For this review, take the finished solid that the model builds, in its own axes (mm). Face numbers are marked on the shaded views. A direction names the side the tool comes from. Give positions to 0.01 mm unless a question says otherwise; leave off trailing zeros. Order: outer loops, then holes, each group sorted by start corner. A loop starts at its lowest first (then second) coordinate and runs counter-clockwise, first axis right, second up. Notation, with made-up numbers: (46.5, 26.5) -> (88.5, 26.5) arc R24 ccw to (88.5, 46.5) -> close; hole circle Ø2 at (33, 20.25). An arc over 180 degrees is marked (long way). One line per item, written item: value. Start each with the question number.
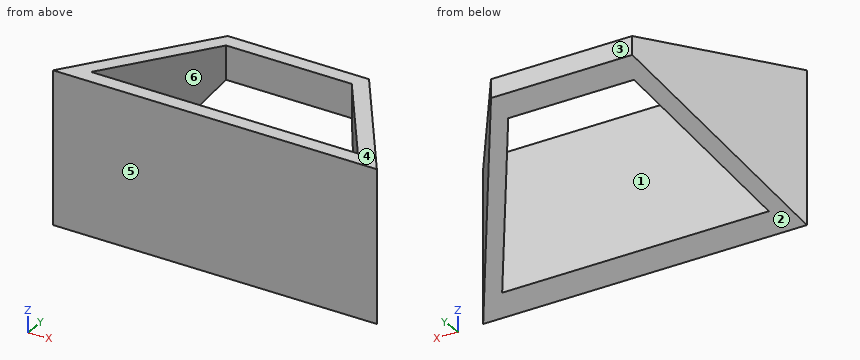
from build123d import *

# Parameters (mm, degrees)
F1_DEPTH      = 1000
F3_DEPTH      = 1091.0655359211
F3_DEPTH_BACK = 1091.0655359211


with BuildPart() as f1:
    # F0 (on Top) → F1 (new body)
    with BuildSketch(Plane.XY):
        Polygon((476.0241719385, 439.0613704803), (-476.0241719385, 439.0613704803), (-1091.0645359211, -439.0613704803), (1091.0645359211, -439.0613704803), align=None)
        Polygon((-898.9354640789, -339.0613704803), (-423.9758280615, 339.0613704803), (423.9758280615, 339.0613704803), (898.9354640789, -339.0613704803), align=None, mode=Mode.SUBTRACT)
    extrude(amount=F1_DEPTH)

    # F2 (on Right) → F3 (cut, two sides)
    with BuildSketch(Plane.YZ) as f3_sk:
        Polygon((-439.0613704803, 0), (439.0613704803, 0), (439.0613704803, 878.1227409606), align=None)
    extrude(amount=-F3_DEPTH, mode=Mode.SUBTRACT)
    extrude(f3_sk.sketch, amount=F3_DEPTH_BACK, mode=Mode.SUBTRACT)


solid = f1.part
Q1. Take a section at B-B (y = -242). State the section outline as (x, z) points, and give its area (3 significant figures).
Q2. For line 1 along Y through (x, z) = (-879.5, 836.5); line 2 along Y through (x, z) = (619, 595.5); line 3 along Y through (x, z) = (-342.5, 617), list the stretches that pass through material, from the lowest coordinate up.
Q3. Mouldability with a two-part tool opening along Y and no side actions: class the marked faces 3, 4, 5 and 6 as pulls with the +Y half, pulls with the -Y half, needs draft (parallel to the pull), parting line crosses it, or undercut.
Q4. Take a section at C-C (z = 430.5). State the section outline as (x, y) points, and give its area (3 significant figures).
Q5. Take a section at A-A (x = -168.5). State the section outline as (y, z) points, and give its area (3 significant figures).
Q6. For pin 1 Ø10 at (y, z) = (-254, 700.5) entering from +X; pin 2 Ø1.5 at (y, z) = (-86, 480) entering from +X; pin 3 Ø8 at (y, z) = (-279, 636.5) entering from +X, all flat-tipped, find the tip position at first contact; note any pin that passes through.
Q7. For the marked faces 1 and 2, list the 3-axis set-ups (+Z, -Z, +X, -X, +Y, -Y) from which the entire face can be reached by the end or side of a thin tool; tool diameter is ignored.
Q8. Take a section at D-D (z = 171.5). State the section outline as (x, y) points, and give its area (3 significant figures).
Answers below:
1. outline: (-953.04, 197.06) -> (-830.95, 197.06) -> (-830.95, 1000) -> (-953.04, 1000) -> close; (830.95, 197.06) -> (953.04, 197.06) -> (953.04, 1000) -> (830.95, 1000) -> close
1. area: 196,000 mm²
2. line 1: y = -439.06 to -339.06, -311.31 to -137
2. line 2: y = -439.06 to -339.06, 60.62 to 156.44
2. line 3: y = -439.06 to -339.06
3. face 3: pulls with the +Y half
3. face 4: needs draft
3. face 5: pulls with the -Y half
3. face 6: undercut
4. outline: (-1091.06, -439.06) -> (1091.06, -439.06) -> (789.54, -8.56) -> (667.45, -8.56) -> (898.94, -339.06) -> (-898.94, -339.06) -> (-667.45, -8.56) -> (-789.54, -8.56) -> close
4. area: 292,000 mm²
5. outline: (-439.06, 0) -> (-339.06, 100) -> (-339.06, 1000) -> (-439.06, 1000) -> close; (339.06, 778.12) -> (439.06, 878.12) -> (439.06, 1000) -> (339.06, 1000) -> close
5. area: 112,000 mm²
6. pin 1: stops at x = 964.95
6. pin 2: stops at x = 844.3
6. pin 3: stops at x = 981.76
7. face 1: +Z, -Z
7. face 2: -Z, +X, -X, +Y
8. outline: (-1091.06, -439.06) -> (1091.06, -439.06) -> (970.95, -267.56) -> (848.86, -267.56) -> (898.94, -339.06) -> (-898.94, -339.06) -> (-848.86, -267.56) -> (-970.95, -267.56) -> close
8. area: 229,000 mm²
